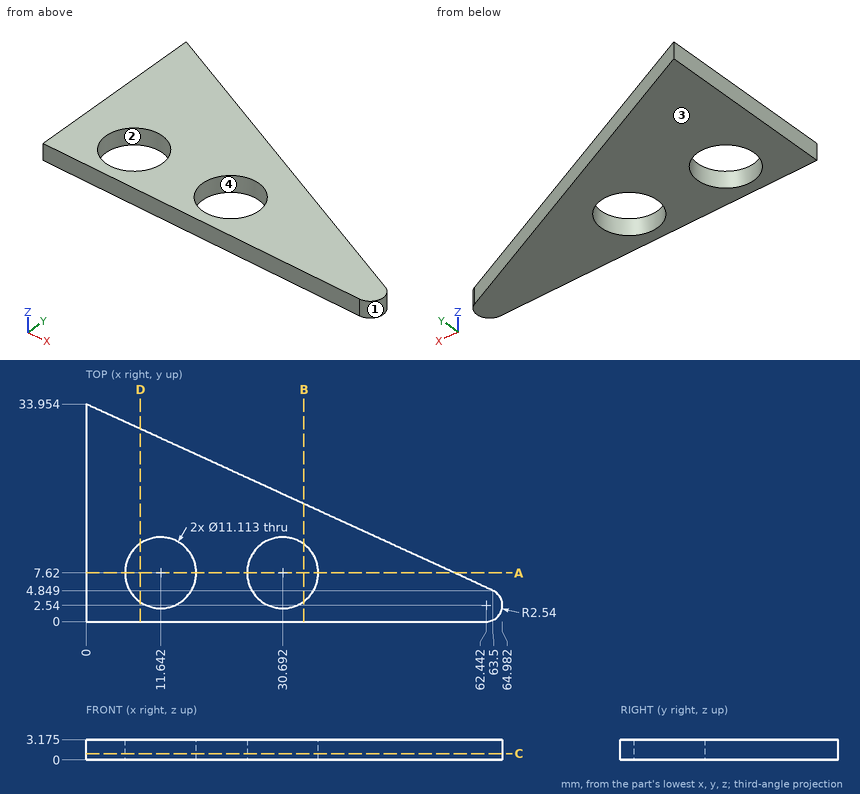
Design review of the part shown in the three views and the two pictorial views. Dimensions are in mm from the part's minimum x, y and z. Round coordinates to 2 decimals unless told otherwise and drop trailing zeros. Loops run counter-clockwise (first coordinate to the right, second up) from the corner with the lowest first, then second, coordinate; pieces in that order, holes last.
1) Consider section D-D on x = 8.5. State the section outline as (y, z) points (1 decimal).
Values follow:
outline: (0, 0) - (3, 0) - (3, 3.2) - (0, 3.2) - close; (12.2, 0) - (30.1, 0) - (30.1, 3.2) - (12.2, 3.2) - close
2) Wall thickness on line 1 along X through (y, z) = (5, 1.1) (1 decimal); line 2 along Y through (x, z) = (26, 0.95) (1 decimal); line 3 along Y through (x, z) = (30, 0.5) (1 decimal): over which ranges is each line inside the solid? List them lowest first.
Values follow:
line 1: x = 0 to 6.7, 16.5 to 25.8, 35.6 to 63.2
line 2: y = 0 to 4.6, 10.6 to 22
line 3: y = 0 to 2.1, 13.1 to 20.2
3) Consider section B-B on x = 34. State the section outline as (y, z) points (1 decimal).
Values follow:
outline: (0, 0) - (3.2, 0) - (3.2, 3.2) - (0, 3.2) - close; (12.1, 0) - (18.4, 0) - (18.4, 3.2) - (12.1, 3.2) - close
4) Clearance check with flat-ended pins moving along their axes: P1, Ø1.5, axis at x = 8, z = 1, coming from the +Y side; P2, Ø1.5, axis at y = 14, z = 2.5, coming from the +X side (1 decimal); P3, Ø1, axis at y = 9, z = 1, coming from the +X side (1 decimal). State where each tip first meets the part, or that it passes through.
Values follow:
P1: stops at y = 30.63
P2: stops at x = 45.2
P3: stops at x = 55.5
5) Consider section C-C on z = 1. Give the number of separate pieces and of enclosed holes in the cut face, then the cut area to 3 significant figures.
Values follow:
separate pieces: 1
enclosed holes: 2
area: 1,040 mm2
6) The part is to be moulded in two halves that separate along Y. For the marked faces 1, 2, 3 and 4, say which applies: pulls with the +Y half, pulls with the -Y half, needs draft (parallel to the pull), parting line crosses it, or undercut.
Values follow:
face 1: parting line crosses it
face 2: undercut
face 3: needs draft
face 4: undercut
7) Consider section A-A on y = 7.62. State the section outline as (x, z) points (1 decimal).
Values follow:
outline: (0, 0) - (6.1, 0) - (6.1, 3.2) - (0, 3.2) - close; (17.2, 0) - (25.1, 0) - (25.1, 3.2) - (17.2, 3.2) - close; (36.2, 0) - (57.5, 0) - (57.5, 3.2) - (36.2, 3.2) - close
